Geometry check sheet. Reference: the model listing, model coordinates, mm. A direction names the side the tool comes from. Give positions to 0.01 mm unless a question says otherwise; leave off trailing zeros. Order: outer loops, then holes, each group sorted by start corner. A loop starts at its lowest first (then second) coordinate and runs counter-clockwise, first axis right, second up.
Autodesk Inventor part; units mm, degrees
ref_plane "YZ Plane" through (0, 0, 0) normal (1, 0, 0) x (0, 1, 0)
ref_plane "XZ Plane" through (0, 0, 0) normal (0, 1, 0) x (-1, 0, 0)
ref_plane "XY Plane" through (0, 0, 0) normal (0, 0, 1) x (1, 0, 0)
sketch "Sketch2" plane through (0, 0, 0) normal (0, 1, 0) x (-1, 0, 0)
  line L0 (150, 10.1481) -> (-142.3178, 10.1481)
  line L1 (-142.3178, -9.8519) -> (150, -9.8519)
  line L2 (150, -9.8519) -> (150, 10.1481)
  line L3 (-142.3178, 10.1481) -> (-142.3178, 210.1481)
  line L4 (-142.3178, 210.1481) -> (-162.3178, 210.1481)
  line L5 (-162.3178, 210.1481) -> (-162.3178, -209.8519)
  line L6 (-162.3178, -209.8519) -> (-142.3178, -209.8519)
  line L7 (-142.3178, -209.8519) -> (-142.3178, -9.8519)
  point P0 (0, 0)
  dimension "d0" = 20
  dimension "d2" = 150
  dimension "d3" = 200
  dimension "d4" = 420
  dimension "d5" = 20
  dimension "d6" = 292.3178
  dimension "d7" = 20
extrude "Extrusion1" add sketch "Sketch2" along normal blind 20
sketch "Sketch3" plane through (142.3178, 0, -209.8519) normal (-1, 0, 0) x (0, 0, 1)
  line L0 (0, 120) -> (20, 120)
  line L1 (20, 120) -> (20, -100)
  line L2 (20, -100) -> (0, -100)
  line L3 (0, -100) -> (0, 120)
  line L4 (0, 0) -> (200, 0)
  line L5 (0, 20) -> (200, 20)
  line L6 (420, -100) -> (400, -100)
  line L7 (400, -100) -> (400, 120)
  line L8 (400, 120) -> (420, 120)
  line L9 (420, 120) -> (420, -100)
  line L10 (420, 0) -> (420, 20)
  line L11 (220, 0) -> (420, 0)
  line L12 (220, 20) -> (420, 20)
  point P0 (209.8519, 0)
  point P1 (400, 20)
  point P2 (400, 0)
  dimension "d10" = 100
  dimension "d11" = 100
  dimension "d12" = 20
  dimension "d13" = 20
  dimension "d14" = 0
  dimension "d15" = 100
  dimension "d16" = 100
extrude "Extrusion2" add sketch "Sketch3" against normal blind 20 contours L0 L1 L5 L3 | L5 L1 L4 L3 | L4 L1 L2 L3 | L6 L7 L11 L9 | L12 L7 L8 L9
sketch "Sketch8" plane through (0, 20, 0) normal (0, 1, 0) x (1, 0, 0)
  line L0 (-150, 9.8519) -> (-150, -10.1481)
  line L1 (-92.5, -2.5) -> (-87.5, -2.5)
  line L2 (-87.5, -2.5) -> (-87.5, 2.5)
  line L3 (-87.5, 2.5) -> (-92.5, 2.5)
  line L4 (-92.5, 2.5) -> (-92.5, -2.5)
  point P0 (0, 0)
  point P1 (-90, 0)
  point P2 (-150, -0.1481)
  point P3 (-90, -2.5)
  point P4 (-87.5, 0)
  dimension "d36" = 60
  dimension "d37" = 2.5
  dimension "d38" = 5
  dimension "d39" = 5
  dimension "d40" = 2.5
extrude "Extrusion4" cut sketch "Sketch8" against normal through all
properties part number "statyw"
Item 1: Sectioned sample at A-A (y = 83). Enter the section's corners in (x, z).
Reported:
outline: (142.32, -209.85) - (162.32, -209.85) - (162.32, -189.85) - (142.32, -189.85) - close; (142.32, 190.15) - (162.32, 190.15) - (162.32, 210.15) - (142.32, 210.15) - close
Item 2: Gauge pin test, flat ends, axial feed: pin 1 (5.5 mm diameter, centred on x = -89, y = 8.5, fed in from -Z); pin 2 (16 mm diameter, centred on x = 52, y = 10, fed in from +Z); pin 3 (10 mm diameter, centred on x = -51, z = 7, fed in from -Y). Record the tip position at first contact, or that the pin passes through.
Reported:
pin 1: stops at z = -9.85
pin 2: stops at z = 10.15
pin 3: stops at y = 0
Item 3: Draft check along Z on faces 1 (the flat face through (152, 69, 190.148)), 2 (the flat face through (152, -49, -189.852)), 3 (the flat face through (162.318, 9, 1)), 4 (the flat face through (-6, 10, 10.148)). Enter one of: released by +Z, released by -Z, zero draft, split by the parting line, or undercut.
Reported:
face 1: undercut
face 2: undercut
face 3: zero draft
face 4: released by +Z
Item 4: Set-up check for faces 5 (the flat face through (99, 20, 1)), 6 (the flat face through (99, 0, 1)), 7 (the flat face through (142.318, 9, 154)), 8 (the flat face through (152, -100, 200)), 9 (the flat face through (142.318, 9, -147)): record each of +Z, -Z, +X, -X, +Y, -Y from which the full face is reachable in a straight line by a thin tool's end or side.
Reported:
face 5: +X, -X, +Y
face 6: +X, -X, -Y
face 7: +Z, -X, +Y, -Y
face 8: +Z, -Z, +X, -X, -Y
face 9: -Z, -X, +Y, -Y
Item 5: Scan lines: L1, parallel to Y at x = -130.5, z = -6; L2, parallel to Z at x = 96, y = 1.5. Record each from-to range of solid material in increasing order.
Reported:
L1: y = 0 to 20
L2: z = -9.85 to 10.15
Item 6: Sectioned sample at B-B (z = 107.5). Enter the section's corners in (x, y), and give its area (3 significant figures).
Reported:
outline: (142.32, 0) - (162.32, 0) - (162.32, 20) - (142.32, 20) - close
area: 400 mm2
Item 7: Sectioned sample at C-C (x = 109). Enter the section's corners in (y, z).
Reported:
outline: (0, -9.85) - (20, -9.85) - (20, 10.15) - (0, 10.15) - close
